Part model, mm, in its own coordinate system. A direction names the side the tool comes from. Round coordinates to 2 decimals unless told otherwise and drop trailing zeros. Loops run counter-clockwise (first coordinate to the right, second up) from the corner with the lowest first, then second, coordinate; pieces in that order, holes last. Notation, with made-up numbers: (11, -33) - (52, -33) arc R32 ccw to (52, -3) - close; hole circle Ø7 at (-17.75, -39). An arc over 180 degrees is marked (long way). Put each result on its own line as item: value.
from build123d import *

# Parameters (mm, degrees)
SKETCH2_W           = 114.3
SKETCH2_H           = 254
BOSS_EXTRUDE1_DEPTH = 19.05
CUT_EXTRUDE1_DEPTH  = 280.1834388


with BuildPart() as part:
    # Sketch2 → Boss-Extrude1 (new body)
    with BuildSketch(Plane(origin=(0, 0, 0), x_dir=(0, 0, -1), z_dir=(1, 0, 0))):
        with Locations((57.15, 127)):
            Rectangle(SKETCH2_W, SKETCH2_H)
    extrude(amount=BOSS_EXTRUDE1_DEPTH)

    # Sketch3 → Cut-Extrude1 (cut, through all)
    with BuildSketch(Plane(origin=(19.05, 0, 0), x_dir=(0, 0, -1), z_dir=(1, 0, 0))):
        with BuildLine():
            Line((73.025, 254), (41.275, 254))
            Line((41.275, 254), (41.275, 228.6))
            ThreePointArc((41.275, 228.6), (57.15, 212.725), (73.025, 228.6))
            Line((73.025, 228.6), (73.025, 254))
        make_face()
    extrude(amount=-CUT_EXTRUDE1_DEPTH, mode=Mode.SUBTRACT)


solid = part.part
1. Pin check, flat tip, straight feed: P1, Ø4, axis at y = 145.5, z = -82.5, coming from the -X side. Stop position of the tip, or through.
A:
P1: stops at x = 0
2. Two-plate mould, pull along Z, no slides. Class faces 3 (the flat face through (9, 125, -114.3)), 4 (the flat face through (9, 125, 0)), 5 (the flat face through (10, 241, -73.025)): pulls with the +Z half, pulls with the -Z half, needs draft (parallel to the pull), parting line crosses it, or undercut.
A:
face 3: pulls with the -Z half
face 4: pulls with the +Z half
face 5: undercut
3. Tool access for faces 1 (the flat face through (10, 241, -41.275)), 2 (the flat face through (19.05, 129, -56)): list every direction of +Z, -Z, +X, -X, +Y, -Y with a clear straight run to the whole face (end or side of a thin tool).
A:
face 1: +X, -X, +Y
face 2: +Z, -Z, +X, +Y, -Y
4. Band-saw the part on B-B (z = -57.15). List the corners of the cut face in (x, y) (3 decimals).
A:
outline: (0, 0) - (19.05, 0) - (19.05, 212.725) - (0, 212.725) - close
5. Band-saw the part on A-A (x = 4). List the corners of the cut face in (y, z) (3 decimals).
A:
outline: (0, -114.3) - (254, -114.3) - (254, -73.025) - (228.6, -73.025) arc R15.875 cw to (228.6, -41.275) - (254, -41.275) - (254, 0) - (0, 0) - close
6. Probe line 1 along Y through (x, z) = (13, -58); line 2 along Z through (x, y) = (7, 215); line 3 along Y through (x, z) = (8, -68). List the from-to ranges inside material, lowest first. Write a range as [from, to].
A:
line 1: y = [0, 212.75]
line 2: z = [-114.3, -65.34], [-48.96, 0]
line 3: y = [0, 217.01]
